from build123d import *

# Parameters (mm, degrees)
BOSS_EXTRUDE1_DEPTH = 8
SKETCH2_R           = 2
CUT_EXTRUDE1_DEPTH  = 25.031021618
SKETCH3_R           = 3
BOSS_EXTRUDE2_DEPTH = 10
FILLET1_R           = 4
FILLET2_R           = 4


with BuildPart() as part:
    # Sketch1 → Boss-Extrude1 (new body)
    with BuildSketch(Plane(origin=(0, 0, 0), x_dir=(1, 0, 0), z_dir=(0, 1, 0))):
        Polygon((1.5, -6.1), (1.5, 6.1), (13.5, 6.1), (13.5, 9.1), (-1.5, 9.1), (-1.5, -9.1), (13.5, -9.1), (13.5, -6.1), align=None)
    extrude(amount=BOSS_EXTRUDE1_DEPTH)

    # Sketch2 → Cut-Extrude1 (cut, through all)
    with BuildSketch(Plane.XY.offset(9.1)):
        with Locations((9.5, 4)):
            Circle(SKETCH2_R)
    extrude(amount=-CUT_EXTRUDE1_DEPTH, mode=Mode.SUBTRACT)

    # Sketch3 → Boss-Extrude2 (add)
    with BuildSketch(Plane.ZY.offset(1.5)):
        with Locations(Location((0, 4, 0), (0, 0, 180))):
            Circle(SKETCH3_R)
    extrude(amount=BOSS_EXTRUDE2_DEPTH)

    # Fillet1
    fillet1_edges = [part.edges().sort_by_distance(p)[0] for p in [
        (13.5, 8, -7.6),
        (13.5, 0, -7.6),
        (13.5, 0, 7.6),
        (13.5, 8, 7.6),
    ]]
    fillet(fillet1_edges, radius=FILLET1_R - 0.0001)  # a hair under: the kernel refuses the full size

    # Fillet2
    fillet2_edges = [part.edges().sort_by_distance(p)[0] for p in [
        (1.5, 4, -6.1),
        (1.5, 4, 6.1),
        (-1.5, 4, 9.1),
        (-1.5, 4, -9.1),
    ]]
    fillet(fillet2_edges, radius=FILLET2_R)


solid = part.part
Model file for the job. Use its own axes, mm. A direction names the side the tool comes from. Coordinates: 2 decimals unless noted, no trailing zeros. Write each loop counter-clockwise with the first axis right and the second up, starting at its lowest first coordinate (ties: lowest second). Pieces come first, ordered by that corner, then holes. Notation, with made-up numbers: (73, -19) -> (82, -19) arc R20 cw to (82, 7) -> close; hole circle Ø5 at (76, -8.75). An arc over 180 degrees is marked (long way). One line per item, written item: value. Start each with the question number.
1) Probe probe 1 along Z at (x, y) = (10.25, 1.5); probe 2 along Y at (x, z) = (9.5, 7.3); probe 3 along X at (y, z) = (6, 0). List the from-to ranges inside material, lowest first.
2) Slice it at B-B on x = 4.5. Write the cut outline in (y, z), then the cut area to 3 significant figures.
3) Slice it at C-C on y = 3.25. Write the cut outline in (x, z).
4) Flat gauge pins, fed straight in: pin 1 Ø2 at (x, y) = (-4, 2) entering from -Z; pin 2 Ø3 at (x, y) = (9.5, 4) entering from -Z; pin 3 Ø1.3 at (y, z) = (2.5, 0.5) entering from +X; pin 4 Ø1.5 at (y, z) = (2, 4) entering from +X. Where does each tip first touch, or does it go through?
5) Slice it at D-D on z = -1.5. Write the cut outline in (x, y), then the cut area to 3 significant figures.
6) Pull direction Y, two halves, no side cores. Call faces 4 (the face through (7, 4, 6.1)), 5 (the face through (9.066, 2.048, 7.621)), 6 (the face through (9.066, 2.048, -7.579)), 7 (the face through (12.297, 1.141, -7.621)): +Y half, -Y half, draft (parallel to the pull), parting line (faces both ways), or undercut.
7) Which spindle directions (+Z, -Z, +X, -X, +Y, -Y) get a long thin tool onto all of the face, cutting with end or side? Do faces 1 (the face through (7, 4, -9.1)), 2 (the face through (1.5, 4, 0)), 3 (the face through (-1.5, 3.9, -3.5)). Say none if no direction does.
Answers follow:
1. probe 1: -9.1 to -6.1, 6.1 to 9.1
1. probe 2: 0 to 2, 6 to 8
1. probe 3: -11.5 to 1.5
2. outline: (0, -9.1) -> (8, -9.1) -> (8, -5.97) -> (0, -5.97) -> close; (0, 5.97) -> (8, 5.97) -> (8, 9.1) -> (0, 9.1) -> close
2. area: 50.0 mm2
3. outline: (-11.5, -2.9) -> (-1.5, -2.9) -> (-1.5, -5.1) arc R4 ccw to (2.5, -9.1) -> (7.65, -9.1) -> (7.65, -6.1) -> (5.5, -6.1) arc R4 cw to (1.5, -2.1) -> (1.5, 2.1) arc R4 cw to (5.5, 6.1) -> (7.65, 6.1) -> (7.65, 9.1) -> (2.5, 9.1) arc R4 ccw to (-1.5, 5.1) -> (-1.5, 2.9) -> (-11.5, 2.9) -> close; (11.35, -9.1) -> (13.43, -9.1) -> (13.43, -6.1) -> (11.35, -6.1) -> close; (11.35, 6.1) -> (13.43, 6.1) -> (13.43, 9.1) -> (11.35, 9.1) -> close
4. pin 1: z = -2.83
4. pin 2: through
4. pin 3: x = 1.5
4. pin 4: x = 2.5
5. outline: (-11.5, 1.4) -> (-1.5, 1.4) -> (-1.5, 0) -> (1.5, 0) -> (1.5, 8) -> (-1.5, 8) -> (-1.5, 6.6) -> (-11.5, 6.6) -> close
5. area: 76.0 mm2
6. face 4: draft
6. face 5: undercut
6. face 6: undercut
6. face 7: -Y half
7. face 1: -Z, +X, -X, +Y, -Y
7. face 2: +X, +Y, -Y
7. face 3: -X
